Read the model definition and answer for the solid it produces. Units are mm, in the model's axes. A direction names the side the tool comes from. Coordinates: 2 decimals unless noted, no trailing zeros. Write each loop counter-clockwise with the first axis right and the second up, starting at its lowest first coordinate (ties: lowest second). Pieces come first, ordered by that corner, then holes. Notation, with made-up numbers: (-3, 21.25) - (29, 21.25) arc R24 cw to (29, 49.25) - close; hole circle Ø7 at (82, 57.5). An arc over 180 degrees is marked (long way). Use a Markdown table: item, result.
from build123d import *

# Parameters (mm, degrees)
SKETCH2_R           = 38.1
BOSS_EXTRUDE1_DEPTH = 158.75
CUT_EXTRUDE1_DEPTH  = 47.625
SKETCH4_R           = 12.7
CUT_EXTRUDE2_DEPTH  = 67.675


with BuildPart() as part:
    # Sketch2 → Boss-Extrude1 (new body, symmetric)
    with BuildSketch(Plane(origin=(0, 0, 0), x_dir=(0, 0, -1), z_dir=(1, 0, 0))):
        Circle(SKETCH2_R)
    extrude(amount=BOSS_EXTRUDE1_DEPTH, both=True)

    # Sketch3 → Cut-Extrude1 (cut)
    with BuildSketch(Plane(origin=(158.75, 0, 0), x_dir=(0, 0, -1), z_dir=(1, 0, 0))):
        with BuildLine():
            Line((-28.575, 25.200781238), (-28.575, -25.200781238))
            ThreePointArc((-28.575, -25.200781238), (-38.1, 0), (-28.575, 25.200781238))
        make_face()
        with BuildLine():
            Line((28.575, 25.200781238), (28.575, -25.200781238))
            ThreePointArc((28.575, -25.200781238), (38.1, 0), (28.575, 25.200781238))
        make_face()
    extrude(amount=-CUT_EXTRUDE1_DEPTH, mode=Mode.SUBTRACT)

    # Sketch4 → Cut-Extrude2 (cut, through all)
    with BuildSketch(Plane.XY.offset(28.575)):
        with Locations((139.7, 0)):
            Circle(SKETCH4_R)
    extrude(amount=-CUT_EXTRUDE2_DEPTH, mode=Mode.SUBTRACT)


solid = part.part
(1) Each of these flat-tipped pins is pushed along its axis until it touches: P1, Ø6, axis at x = -63, y = 21, coming from the +Z side; P2, Ø1, axis at x = -65, y = -8.5, coming from the -Z side; P3, Ø4, axis at x = 75, y = 2, coming from the +Z side; P4, Ø23, axis at x = 139.7, y = 0, coming from the +Z side. Where does it stop, or does it pass through?
Report:
| item | result |
|---|---|
| P1 | stops at z = 33.58 |
| P2 | stops at z = -37.25 |
| P3 | stops at z = 38.1 |
| P4 | passes through |
(2) Straight lines are drawn through the part: L1, parallel to X at y = 1, z = -21.5; L2, parallel to Y at x = 139.7, z = 1.5; L3, parallel to Y at x = 139.7, z = 12. For each, find the intervals that lie inside material, in ascending order.
Report:
| item | result |
|---|---|
| L1 | x = -158.75 to 127.04, 152.36 to 158.75 |
| L2 | y = -38.07 to -12.7, 12.7 to 38.07 |
| L3 | y = -36.16 to -12.7, 12.7 to 36.16 |
(3) For faces 1 (the flat face through (158.75, 1, 0)), 2 (the flat face through (111.125, 0, 32)), 3 (the flat face through (125, 0, -28.575)), determine the directions among +Z, -Z, +X, -X, +Y, -Y from which every point of the face is accessible in a straight line to the end or side of a thin tool.
Report:
| item | result |
|---|---|
| face 1 | +Z, -Z, +X, +Y, -Y |
| face 2 | +Z, +X, +Y, -Y |
| face 3 | -Z, +X, +Y, -Y |
(4) A cutting plane is placed at C-C, the plane z = 0. Write down the section's boundary in (x, y).
Report:
| item | result |
|---|---|
| outline | (-158.75, -38.1) - (158.75, -38.1) - (158.75, 38.1) - (-158.75, 38.1) - close; hole circle Ø25.4 at (139.7, 0) |
(5) A cutting plane is placed at A-A, the plane x = 139.7. Write down the section's boundary in (y, z) (3 decimals).
Report:
| item | result |
|---|---|
| outline | (-25.201, -28.575) - (-12.7, -28.575) - (-12.7, 28.575) - (-25.201, 28.575) arc R38.1 ccw to start; (12.7, -28.575) - (25.201, -28.575) arc R38.1 ccw to (25.201, 28.575) - (12.7, 28.575) - close |
(6) A cutting plane is placed at B-B, the plane y = 0. Write down the section's boundary in (x, z) (3 decimals), and give its area (3 significant figures).
Report:
| item | result |
|---|---|
| outline | (-158.75, -38.1) - (111.125, -38.1) - (111.125, -28.575) - (127, -28.575) - (127, 28.575) - (111.125, 28.575) - (111.125, 38.1) - (-158.75, 38.1) - close; (152.4, -28.575) - (158.75, -28.575) - (158.75, 28.575) - (152.4, 28.575) - close |
| area | 21,800 mm² |
(7) A cutting plane is placed at D-D, the plane x = -114. Write down the section's boundary in (y, z), and give its area (3 significant figures).
Report:
| item | result |
|---|---|
| outline | circle Ø76.2 at (0, 0) |
| area | 4,560 mm² |
(8) The mould has two halves that part along Y. Classify faces 4 (the cylindrical face through (2.222, 37.776, 4.96)), 5 (the cylindrical face through (151.814, 3.815, 0.4)), 6 (the flat face through (-158.75, 1, 1)): pulls with the +Y half, pulls with the -Y half, needs draft (parallel to the pull), parting line crosses it, or undercut.
Report:
| item | result |
|---|---|
| face 4 | parting line crosses it |
| face 5 | undercut |
| face 6 | needs draft |
